```python
from build123d import *

# Parameters (mm, degrees)
SKETCH1_W           = 292.1
SKETCH1_H           = 292.1
BOSS_EXTRUDE1_DEPTH = 6.35
SKETCH3_W           = 25.4
SKETCH3_H           = 6.35
BOSS_EXTRUDE2_DEPTH = 6.35
SKETCH4_W           = 25.4
SKETCH4_H           = 6.35
BOSS_EXTRUDE3_DEPTH = 6.35
SKETCH5_R           = 3.25
SKETCH5_W           = 86.36
SKETCH5_H           = 86.36
CUT_EXTRUDE1_DEPTH  = 6.35


with BuildPart() as part:
    # Sketch1 → Boss-Extrude1 (new body)
    with BuildSketch(Plane(origin=(0, 0, 0), x_dir=(1, 0, 0), z_dir=(0, 1, 0))):
        with Locations((-8.203162495, -54.546418503)):
            Rectangle(SKETCH1_W, SKETCH1_H)
    extrude(amount=BOSS_EXTRUDE1_DEPTH)

    # Sketch3 → Boss-Extrude2 (add)
    with BuildSketch(Plane.ZY.offset(154.253162495)):
        with Locations((-40.703581497, 3.175)):
            Rectangle(SKETCH3_W, SKETCH3_H)
        with Locations((149.796418503, 3.175)):
            Rectangle(SKETCH3_W, SKETCH3_H)
        with Locations((54.546418503, 3.175)):
            Rectangle(SKETCH3_W, SKETCH3_H)
    boss_extrude2 = extrude(amount=BOSS_EXTRUDE2_DEPTH)

    # Mirror1: Boss-Extrude2 across plane
    add(boss_extrude2.mirror(Plane.ZY.offset(8.203162495)))

    # Sketch4 → Boss-Extrude3 (add)
    with BuildSketch(Plane(origin=(0, 0, -91.503581497), x_dir=(-1, 0, 0), z_dir=(0, 0, -1))):
        with Locations((-93.396837505, 3.175)):
            Rectangle(SKETCH4_W, SKETCH4_H)
        with Locations((109.803162495, 3.175)):
            Rectangle(SKETCH4_W, SKETCH4_H)
        with Locations((8.203162495, 3.175)):
            Rectangle(SKETCH4_W, SKETCH4_H)
    boss_extrude3 = extrude(amount=BOSS_EXTRUDE3_DEPTH)

    # Mirror2: Boss-Extrude3 across plane
    add(boss_extrude3.mirror(Plane.XY.offset(54.546418503)))

    # Sketch5 → Cut-Extrude1 (cut)
    with BuildSketch(Plane.XZ):
        with Locations(Location((-8.203162495, 118.046418503, 0), (0, 0, 270))):
            Circle(SKETCH5_R)
        with Locations(Location((55.296837505, 54.546418503, 0), (0, 0, 270))):
            Circle(SKETCH5_R)
        with Locations(Location((-8.203162495, -8.953581497, 0), (0, 0, 270))):
            Circle(SKETCH5_R)
        with Locations(Location((-71.703162495, 54.546418503, 0), (0, 0, 270))):
            Circle(SKETCH5_R)
        with Locations((-8.203162495, 54.546418503)):
            Rectangle(SKETCH5_W, SKETCH5_H)
        Polygon((106.096837505, 200.596418503), (137.846837505, 162.496418503), (137.846837505, 200.596418503), align=None)
        Polygon((-122.503162495, 200.596418503), (-154.253162495, 200.596418503), (-154.253162495, 162.496418503), align=None)
        Polygon((-154.253162495, -53.403581497), (-154.253162495, -91.503581497), (-122.503162495, -91.503581497), align=None)
        Polygon((106.096837505, -91.503581497), (137.846837505, -91.503581497), (137.846837505, -53.403581497), align=None)
    extrude(amount=-CUT_EXTRUDE1_DEPTH, mode=Mode.SUBTRACT)


solid = part.part
```
Geometry: final body of the model. Coordinates: model frame, mm. Give positions to 0.01 mm unless a question says otherwise; leave off trailing zeros. Loops run counter-clockwise (first coordinate to the right, second up) from the corner with the lowest first, then second, coordinate; pieces in that order, holes last. Notation, with made-up numbers: (76.25, -2) -> (101.25, -2) arc R27 ccw to (101.25, 15) -> close; hole circle Ø1 at (7, 68.5). An arc over 180 degrees is marked (long way). Return JSON: item names as keys, results as strings.
Item 1: Line query: line 1 (X direction, y = 4, z = 33); line 2 (Z direction, x = -30, y = 2.75); line 3 (X direction, y = 3, z = 60). Output: solid intervals per line, ascending.
Filled in:
{"line 1": "-154.25 to -51.38, 34.98 to 137.85", "line 2": "-91.5 to 11.37, 97.73 to 200.6", "line 3": "-160.6 to -51.38, 34.98 to 144.2"}
Item 2: Pin query (flat end, axial travel): P1, Ø1.9, axis at y = 2.5, z = 205, coming from the +X side; P2, Ø3, axis at x = 139.5, y = 3.5, coming from the -Z side; P3, Ø1.9, axis at y = 2.5, z = -95, coming from the -X side. Return the tip coordinate at first contact, or that it passes through.
Filled in:
{"P1": "x = 106.1", "P2": "z = -53.4", "P3": "x = -122.5"}
Item 3: Section D-D, the plane y = 2.75. Count the separate pieces of the cut face and the enclosed holes in it, plus the area to 3 significant figures.
Filled in:
{"separate pieces": "1", "enclosed holes": "5", "area": "77,200 mm^2"}
Item 4: Section C-C, the plane x = 69.5. Output: boundary loops of the cut face in (y, z), plus the area to 3 significant figures.
Filled in:
{"outline": "(0, -91.5) -> (6.35, -91.5) -> (6.35, 200.6) -> (0, 200.6) -> close", "area": "1,850 mm^2"}
Item 5: Section B-B, the plane x = -39.5. Output: boundary loops of the cut face in (y, z), plus the area to 3 significant figures.
Filled in:
{"outline": "(0, -91.5) -> (6.35, -91.5) -> (6.35, 11.37) -> (0, 11.37) -> close; (0, 97.73) -> (6.35, 97.73) -> (6.35, 200.6) -> (0, 200.6) -> close", "area": "1,310 mm^2"}
Item 6: Section A-A, the plane z = 81. Output: boundary loops of the cut face in (x, y).
Filled in:
{"outline": "(-154.25, 0) -> (-51.38, 0) -> (-51.38, 6.35) -> (-154.25, 6.35) -> close; (34.98, 0) -> (137.85, 0) -> (137.85, 6.35) -> (34.98, 6.35) -> close"}
Item 7: Mould query, pull axis Z, two halves, no side actions, for faces 1 (the flat face through (-10, 0, -15)), 2 (the cylindrical face through (-5.46, 3.13, -10.7)), 3 (the flat face through (121.75, 3.13, 181.81)), 4 (the flat face through (122.19, 3.13, -72.19)). Classes: released by +Z, released by -Z, zero draft, split by the parting line, or undercut.
Filled in:
{"face 1": "zero draft", "face 2": "undercut", "face 3": "released by +Z", "face 4": "released by -Z"}
